Autodesk Inventor part; units mm, degrees
ref_plane "YZ Plane" through (0, 0, 0) normal (1, 0, 0) x (0, 1, 0)
ref_plane "XZ Plane" through (0, 0, 0) normal (0, 1, 0) x (-1, 0, 0)
ref_plane "XY Plane" through (0, 0, 0) normal (0, 0, 1) x (1, 0, 0)
sketch "Sketch1" plane through (0, 0, 0) normal (0, 0, 1) x (1, 0, 0)
  line L0 (-38.2565, 12.5) -> (25.2435, 12.5)
  line L1 (25.2435, 12.5) -> (25.2435, -139.9)
  line L2 (25.2435, -139.9) -> (-38.2565, -139.9)
  line L3 (-38.2565, -139.9) -> (-38.2565, 12.5)
  point P0 (0, 0)
  dimension "d0" = 63.5
  dimension "d1" = 152.4
extrude "Extrusion1" add sketch "Sketch1" along normal blind 114.3
sketch "Sketch2" plane through (0, 0, 114.3) normal (0, 0, 1) x (1, 0, 0)
  line L0 (-38.2565, -139.9) -> (-38.2565, 12.5)
  line L1 (25.2435, -139.9) -> (-38.2565, -139.9)
  line L2 (-38.2565, -7.0772) -> (25.2435, -7.0772)
  line L3 (25.2435, -7.0772) -> (25.2435, -139.9)
  line L4 (25.2435, -139.9) -> (-38.2565, -139.9)
  line L5 (-38.2565, -139.9) -> (-38.2565, -7.0772)
  point P0 (0, 0)
extrude "Extrusion2" cut sketch "Sketch2" against normal blind 6.35
sketch "Sketch3" plane through (0, 0, 0) normal (0, 0, -1) x (-1, 0, 0)
  line L0 (38.2565, 12.5) -> (-25.2435, 12.5)
  line L1 (-25.2435, 12.5) -> (-25.2435, -139.9)
  line L2 (-25.2435, -139.9) -> (38.2565, -139.9)
  line L3 (38.2565, -139.9) -> (38.2565, 12.5)
  point P0 (0, 0)
extrude "Extrusion3" cut sketch "Sketch3" against normal blind 6.35
properties part number "battery"
Could you check a few things on this model? Use its own coordinates, in mm. A direction names the side the tool comes from. Coordinates: 2 decimals unless noted, no trailing zeros. Write each loop counter-clockwise with the first axis right and the second up, starting at its lowest first coordinate (ties: lowest second). Pieces come first, ordered by that corner, then holes. Notation, with made-up numbers: (-26, 3) -> (4, 3) arc R24 cw to (4, 24) -> close; hole circle Ø3 at (26.25, 62). An arc over 180 degrees is marked (long way). Write item = value, one per line. Start each with the question number.
(1) Will these pins go through, and if not, where does the flat tip stop? pin 1 (5 mm diameter, centred on x = -19, z = 110, fed in from -Y); pin 2 (19 mm diameter, centred on x = -13, y = -64.5, fed in from +Z).
(2) I need wall thicknesses on line 1 (Z direction, x = -28.5, y = -64.5). Which ranges of the line are inside material? Lowest first, please. Write a range as [from, to].
(3) I want a section at A-A (y = -101.5). Please give me the cut outline in (x, z), plus the area to 3 significant figures.
(4) I want a section at B-B (x = 7). Please give me the cut outline in (y, z), plus the area to 3 significant figures.
(5) Which directions (+Z, -Z, +X, -X, +Y, -Y) give clear straight access to the entire face, cutting with the end or side of a thin tool? Please do faces 1 (the face through (-7, -7.077, 111)), 2 (the face through (-6, -63, 6.35)).
Result set:
q1.pin_1 = -139.9
q1.pin_2 = 107.95
q2.line_1 = [6.35, 107.95]
q3.outline = (-38.26, 6.35) -> (25.24, 6.35) -> (25.24, 107.95) -> (-38.26, 107.95) -> close
q3.area = 6,450 mm2
q4.outline = (-139.9, 6.35) -> (12.5, 6.35) -> (12.5, 114.3) -> (-7.08, 114.3) -> (-7.08, 107.95) -> (-139.9, 107.95) -> close
q4.area = 15,600 mm2
q5.face_1 = +Z, +X, -X, -Y
q5.face_2 = -Z, +X, -X, +Y, -Y
